For this review, take the finished solid that the model builds, in its own axes (mm). Face numbers are marked on the shaded views. Coordinates: 2 decimals unless noted, no trailing zeros. Order: outer loops, then holes, each group sorted by start corner. A loop starts at its lowest first (then second) coordinate and runs counter-clockwise, first axis right, second up.
Autodesk Inventor part; units mm, degrees
ref_plane "YZ Plane" through (0, 0, 0) normal (1, 0, 0) x (0, 1, 0)
ref_plane "XZ Plane" through (0, 0, 0) normal (0, 1, 0) x (-1, 0, 0)
ref_plane "XY Plane" through (0, 0, 0) normal (0, 0, 1) x (1, 0, 0)
sketch "Skizze1" plane through (0, 0, 0) normal (0, 0, 1) x (1, 0, 0)
  circle A0 centre (6, 15) radius 2.5
  circle A1 centre (11, 15) radius 0.7835
  line L0 (0, 0) -> (15, 0)
  line L1 (15, 0) -> (15, 30)
  line L2 (0, 30) -> (15, 30)
  line L3 (0, 0) -> (0, 30)
  line L4 (2, 0) -> (2, 30)
extrude "Extrusion1" add sketch "Skizze1" along normal blind 2 contours L4 L2 L1 L0
chamfer "Fasen1" distance 1.7 angle 45 1 edges at (10.2165, 15, 2)
properties part number "LagerHO" material "Polyethylen, hohe Dichte, Gleitfläche"
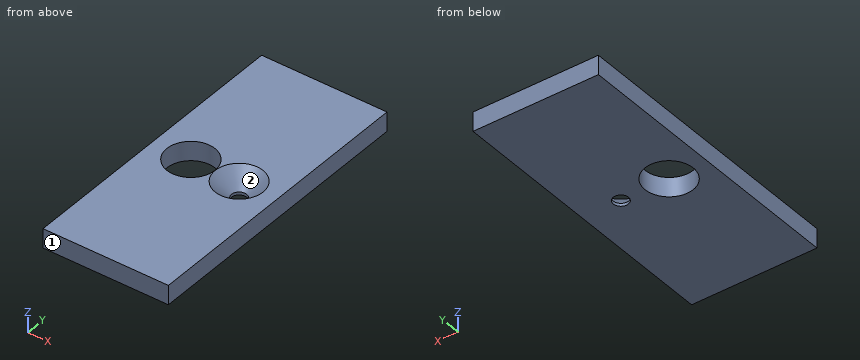
1. Take a section at B-B, the plane x = 11. Give the boundary of the cut face in (y, z).
Answer below:
outline: (0, 0) - (14.22, 0) - (14.22, 0.3) - (12.52, 2) - (0, 2) - close; (15.78, 0) - (30, 0) - (30, 2) - (17.48, 2) - (15.78, 0.3) - close
2. Take a section at A-A, the plane x = 6. Give the boundary of the cut face in (y, z), plus the area to 3 significant figures.
Answer below:
outline: (0, 0) - (12.5, 0) - (12.5, 2) - (0, 2) - close; (17.5, 0) - (30, 0) - (30, 2) - (17.5, 2) - close
area: 50.0 mm2
3. Take a section at C-C, the plane z = 1.2. Give the boundary of the cut face in (x, y).
Answer below:
outline: (2, 0) - (15, 0) - (15, 30) - (2, 30) - close; hole circle Ø5 at (6, 15); hole circle Ø3.37 at (11, 15)
4. Clearance check with a flat-ended pin moving along its axis: pin 1 Ø2 at (x, y) = (4.5, 7) entering from -Z. State where the tip first meets the part, or that it passes through.
Answer below:
pin 1: stops at z = 0
5. To check wall thickness, follow L1, parallel to Y at x = 5.75, z = 0.8; L2, parallel to X at y = 14, z = 0.9; L3, parallel to Y at x = 6.5, z = 1.55. State the ranges of each line that lie inside material, in increasing order.
Answer below:
L1: y = 0 to 12.51, 17.49 to 30
L2: x = 2 to 3.71, 8.29 to 10.04, 11.96 to 15
L3: y = 0 to 12.55, 17.45 to 30
6. The part is to be moulded in two halves that separate along X. For the marked faces 1 and 2, say which applies: +X half, -X half, draft (parallel to the pull), parting line (faces both ways), or undercut.
Answer below:
face 1: draft
face 2: undercut
